Build history of the part. All positions in model axes, mm. A direction names the side the tool comes from. Give positions to 0.01 mm unless a question says otherwise; leave off trailing zeros. Order: outer loops, then holes, each group sorted by start corner. A loop starts at its lowest first (then second) coordinate and runs counter-clockwise, first axis right, second up. Notation, with made-up numbers: (48, 15) -> (59, 15) arc R14 cw to (59, 22) -> close; hole circle Ø8 at (80, -30.75). An arc over 180 degrees is marked (long way). One line per question, with ' | ' between items. Start each with the question number.
(1) Drill centre lines: L1, parallel to Y at x = 47.1, z = -15; L2, parallel to X at y = 9, z = -9.5; L3, parallel to Z at x = -4, y = 2.75. Where is each one in solid material? Low to high. Write a range as from..to.
(2) Pin check, flat tips, straight feed: pin 1 Ø5 at (x, y) = (14.5, 3) entering from -Z; pin 2 Ø4 at (y, z) = (7.5, -15) entering from -X. Stop position of each tip, or through.
(3) Pull direction X, two halves, no side cores. Call faces 1 (the face through (-1, 7, 2.5)), 2 (the face through (-1, 7, -2.5)), 3 (the face through (50, 7, -10)): +X half, -X half, draft (parallel to the pull), parting line (faces both ways), or undercut.
(4) Cut at A-A (y = 7.5). Give the cut face in (x, z).
(5) Cut at C-C (y = 1.5). Give the cut face in (x, z), then the cut area to 3 significant figures.
(6) Cut at B-B (z = -11.5). Give the cut face in (x, y).
(7) Which spindle directions (+Z, -Z, +X, -X, +Y, -Y) get a long thin tool onto all of the face, cutting with end or side? Do faces 4 (the face through (45, 7, -12)), 5 (the face through (0, 15, -1)). Say none if no direction does.
(8) Cut at D-D (z = -16.25). Give the cut face in (x, y), then the cut area to 3 significant figures.
from build123d import *

# Parameters (mm, degrees)
SKETCH1_W           = 100
SKETCH1_H           = 5
SKETCH1_W_2         = 5
SKETCH1_H_2         = 20
BOSS_EXTRUDE1_DEPTH = 15
SKETCH2_R           = 2.5
CUT_EXTRUDE1_DEPTH  = 104.591746776


with BuildPart() as part:
    # Sketch1 → Boss-Extrude1 (new body)
    with BuildSketch(Plane(origin=(0, 0, 0), x_dir=(1, 0, 0), z_dir=(0, 1, 0))):
        Rectangle(SKETCH1_W, SKETCH1_H)
        with Locations((-47.5, 12.5)):
            Rectangle(SKETCH1_W_2, SKETCH1_H_2)
        with Locations((47.5, 12.5)):
            Rectangle(SKETCH1_W_2, SKETCH1_H_2)
    extrude(amount=BOSS_EXTRUDE1_DEPTH)

    # Sketch2 → Cut-Extrude1 (cut, through all)
    with BuildSketch(Plane.ZY.offset(50)):
        with Locations((-15, 7.5)):
            Circle(SKETCH2_R)
    extrude(amount=-CUT_EXTRUDE1_DEPTH, mode=Mode.SUBTRACT)


solid = part.part
Result set:
1) L1: y = 0..5, 10..15 | L2: x = -50..-45, 45..50 | L3: z = -2.5..2.5
2) pin 1: stops at z = -2.5 | pin 2: passes through
3) face 1: draft | face 2: undercut | face 3: +X half
4) outline: (-50, -22.5) -> (-45, -22.5) -> (-45, -17.5) -> (-50, -17.5) -> close; (-50, -12.5) -> (-45, -12.5) -> (-45, -2.5) -> (45, -2.5) -> (45, -12.5) -> (50, -12.5) -> (50, 2.5) -> (-50, 2.5) -> close; (45, -22.5) -> (50, -22.5) -> (50, -17.5) -> (45, -17.5) -> close
5) outline: (-50, -22.5) -> (-45, -22.5) -> (-45, -2.5) -> (45, -2.5) -> (45, -22.5) -> (50, -22.5) -> (50, 2.5) -> (-50, 2.5) -> close | area: 700 mm2
6) outline: (-50, 0) -> (-45, 0) -> (-45, 15) -> (-50, 15) -> close; (45, 0) -> (50, 0) -> (50, 15) -> (45, 15) -> close
7) face 4: -Z, +Y, -Y | face 5: +Z, -Z, +X, -X, +Y
8) outline: (-50, 0) -> (-45, 0) -> (-45, 5.33) -> (-50, 5.33) -> close; (-50, 9.67) -> (-45, 9.67) -> (-45, 15) -> (-50, 15) -> close; (45, 0) -> (50, 0) -> (50, 5.33) -> (45, 5.33) -> close; (45, 9.67) -> (50, 9.67) -> (50, 15) -> (45, 15) -> close | area: 107 mm2
